Can you work these out from the drawing? Everything is in mm from the part's minimum corner. Give positions to 0.01 mm unless a question says otherwise; leave off trailing zeros. Order: outer loops, then holes, each group sorted by start corner. A loop starts at its lowest first (then second) coordinate and runs counter-clockwise, first axis right, second up. Notation, with made-up numbers: (89, 25.25) - (129, 25.25) arc R11 ccw to (129, 42.25) - close; hole circle Ø5 at (16.5, 47.25). An arc over 180 degrees is marked (long way). One line per question, with ' | ' between items.
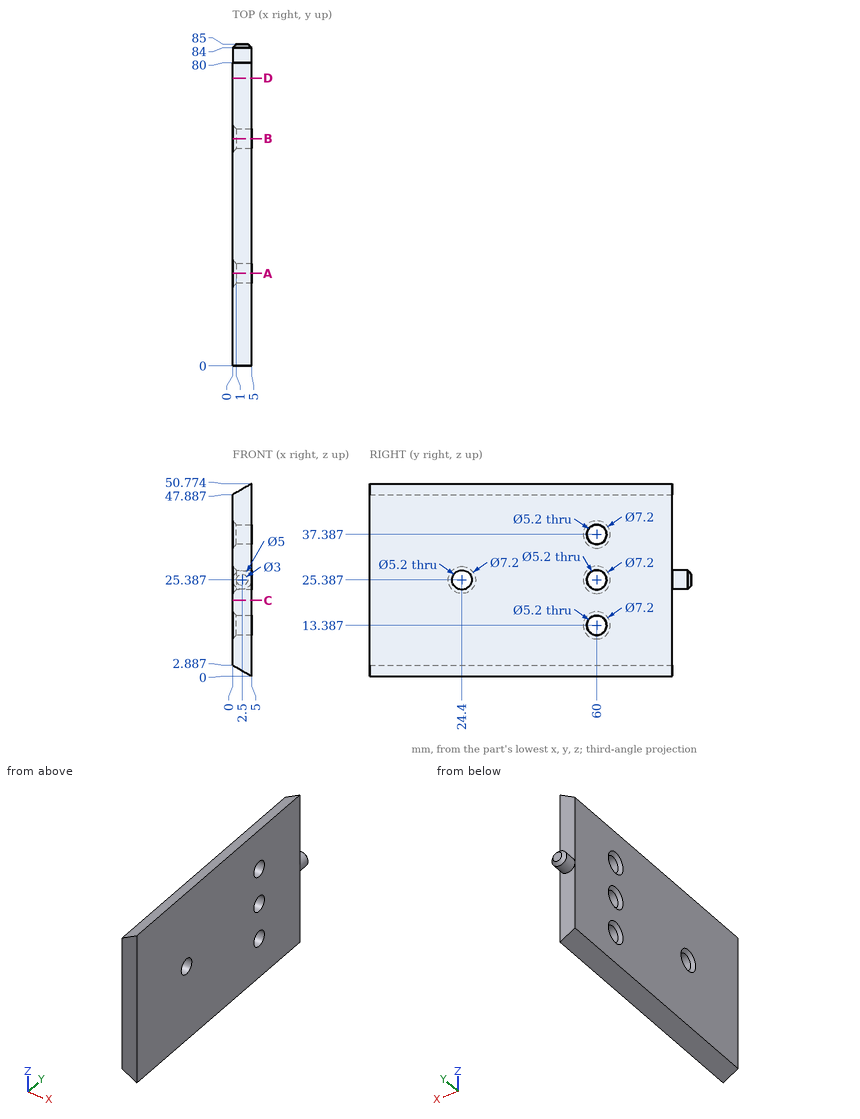
(1) Will these pins go through, and if not, where does the flat tip stop? pin 1 (4.5 mm diameter, centred on y = 24.4, z = 25.39, fed in from +X); pin 2 (1.5 mm diameter, centred on x = 2, z = 22, fed in from +Y); pin 3 (1 mm diameter, centred on x = 3.5, y = 41, fed in from -Z); pin 4 (3 mm diameter, centred on x = 4, y = 58, fed in from -Z).
Answer below:
pin 1: through | pin 2: y = 80 | pin 3: z = 0.58 | pin 4: z = 0
(2) If I drill on line 1 (Z direction, x = 2.55, y = 60) (1 decimal); line 2 (Y direction, x = 4.5, z = 23) (1 decimal); line 3 (Y direction, x = 4.8, z = 6), over which ranges is the centre line in solid material (lowest first)?
Answer below:
line 1: 1.4 to 10.8, 16 to 22.8, 28 to 34.8, 40 to 49.4 | line 2: 0 to 23.4, 25.4 to 59, 61 to 80 | line 3: 0 to 80
(3) Imagine slicing it at A-A (y = 24.4). List the corners of the cut face in (x, z) for me.
Answer below:
outline: (0, 2.89) - (5, 0) - (5, 22.79) - (1, 22.79) - (0, 21.79) - close; (0, 28.99) - (1, 27.99) - (5, 27.99) - (5, 50.77) - (0, 47.89) - close
(4) Imagine slicing it at D-D (y = 76). List the corners of the cut face in (x, z) for me.
Answer below:
outline: (0, 2.89) - (5, 0) - (5, 50.77) - (0, 47.89) - close
(5) Imagine slicing it at B-B (y = 60). List the corners of the cut face in (x, z) for me.
Answer below:
outline: (0, 2.89) - (5, 0) - (5, 10.79) - (1, 10.79) - (0, 9.79) - close; (0, 16.99) - (1, 15.99) - (5, 15.99) - (5, 22.79) - (1, 22.79) - (0, 21.79) - close; (0, 28.99) - (1, 27.99) - (5, 27.99) - (5, 34.79) - (1, 34.79) - (0, 33.79) - close; (0, 40.99) - (1, 39.99) - (5, 39.99) - (5, 50.77) - (0, 47.89) - close
(6) Imagine slicing it at C-C (z = 20). List the corners of the cut face in (x, y) for me.
Answer below:
outline: (0, 0) - (5, 0) - (5, 80) - (0, 80) - close
